Build history of the part. All positions in model axes, mm. Face numbers are marked on the shaded views. A direction names the side the tool comes from. Round coordinates to 2 decimals unless told otherwise and drop trailing zeros. Loops run counter-clockwise (first coordinate to the right, second up) from the corner with the lowest first, then second, coordinate; pieces in that order, holes last. Notation, with made-up numbers: (-9, 9) -> (11, 9) arc R26 ccw to (11, 42) -> close; hole circle Ø11 at (-8.5, 78). An arc over 180 degrees is marked (long way). Put each result on its own line as item: value. Start each with the question number.
Item 1: Drill centre lines: probe 1 along Z at (x, y) = (2.25, 2); probe 2 along Y at (x, z) = (5.25, -16); probe 3 along Y at (x, z) = (5.5, -8). Where is each one in solid material? Low to high. Write a range as [from, to].
Item 2: Cut at D-D, the plane z = 0. List the corners of the cut face in (x, y) (3 decimals).
Item 3: Pull direction Z, two halves, no side cores. Call the marked faces 1, 2 and 3: +Z half, -Z half, draft (parallel to the pull), parting line (faces both ways), or undercut.
Item 4: Cut at A-A, the plane y = 0. List the corners of the cut face in (x, z) (3 decimals).
Item 5: Cut at B-B, the plane z = 9. List the corners of the cut face in (x, y) (3 decimals).
Item 6: Cut at C-C, the plane x = 13.75. List the corners of the cut face in (y, z), plus the area to 3 significant figures.
Item 7: Flat gauge pins, fed straight in: pin 1 Ø9 at (y, z) = (18.02, -17.38) entering from +X (3 decimals); pin 2 Ø11 at (y, z) = (-18.51, 18.23) entering from -X; pin 3 Ø12 at (y, z) = (-20.5, -18.5) entering from +X (3 decimals). Where does each tip first touch, or does it go through?
Item 8: Tool access for the marked faces 4 and 5: list every direction of +Z, -Z, +X, -X, +Y, -Y with a clear straight run to the whole face (end or side of a thin tool).
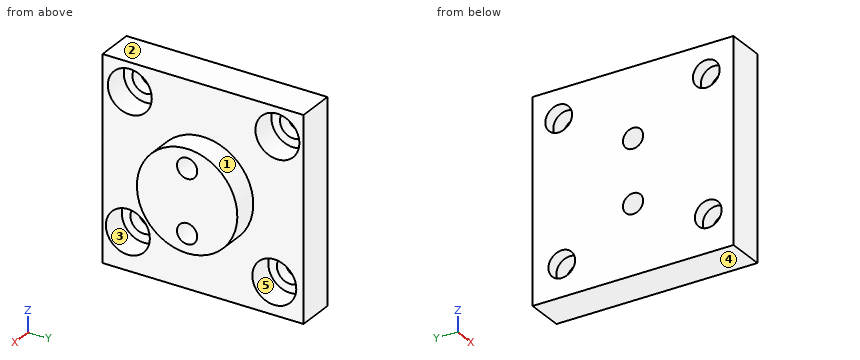
```python
from build123d import *

# Parameters (mm, degrees)
SKETCH1_W                                        = 50.8
SKETCH1_H                                        = 50.8
BOSS_EXTRUDE1_DEPTH                              = 9.525
SKETCH2_R                                        = 12.7
BOSS_EXTRUDE2_DEPTH                              = 6.35
F_1_4_20_TAPPED_HOLE1_D                          = 5.1054
CBORE_FOR_1_4_SOCKET_HEAD_CAP_SCREW1_D           = 6.7564
CBORE_FOR_1_4_SOCKET_HEAD_CAP_SCREW1_CBORE_D     = 11.1125
CBORE_FOR_1_4_SOCKET_HEAD_CAP_SCREW1_CBORE_DEPTH = 6.35


with BuildPart() as part:
    # Sketch1 → Boss-Extrude1 (new body)
    with BuildSketch(Plane(origin=(0, 0, 0), x_dir=(0, 0, -1), z_dir=(1, 0, 0))):
        Rectangle(SKETCH1_W, SKETCH1_H)
    extrude(amount=BOSS_EXTRUDE1_DEPTH)

    # Sketch2 → Boss-Extrude2 (add)
    with BuildSketch(Plane(origin=(9.525, 0, 0), x_dir=(0, 0, -1), z_dir=(1, 0, 0))):
        Circle(SKETCH2_R)
    extrude(amount=BOSS_EXTRUDE2_DEPTH)

    # 1/4-20 Tapped Hole1 (through all)
    with Locations(Plane(origin=(15.875, 0, 0), x_dir=(0, 0, -1), z_dir=(1, 0, 0))):
        with Locations((-7.9375, 0), (7.9375, 0)):
            Hole(F_1_4_20_TAPPED_HOLE1_D / 2)

    # CBORE for 1/4 Socket Head Cap Screw1 (through all)
    with Locations(Plane(origin=(9.525, 0, 0), x_dir=(0, 0, -1), z_dir=(1, 0, 0))):
        with Locations((-18.22919312, 18.79663882), (17.378024569, 18.016400982), (15.959410319, -19.009430957), (-18.22919312, -18.51291597)):
            CounterBoreHole(CBORE_FOR_1_4_SOCKET_HEAD_CAP_SCREW1_D / 2, CBORE_FOR_1_4_SOCKET_HEAD_CAP_SCREW1_CBORE_D / 2, CBORE_FOR_1_4_SOCKET_HEAD_CAP_SCREW1_CBORE_DEPTH)


solid = part.part
```
Reply:
1. probe 1: z = [-25.4, -9.52], [-6.35, 6.35], [9.52, 25.4]
1. probe 2: y = [-25.4, -24.57], [-13.45, 12.63], [23.4, 25.4]
1. probe 3: y = [-25.4, -2.55], [2.55, 25.4]
2. outline: (0, -25.4) -> (9.525, -25.4) -> (9.525, -12.7) -> (15.875, -12.7) -> (15.875, 12.7) -> (9.525, 12.7) -> (9.525, 25.4) -> (0, 25.4) -> close
3. face 1: parting line
3. face 2: +Z half
3. face 3: undercut
4. outline: (0, -25.4) -> (9.525, -25.4) -> (9.525, -12.7) -> (15.875, -12.7) -> (15.875, -10.49) -> (0, -10.49) -> close; (0, -5.385) -> (15.875, -5.385) -> (15.875, 5.385) -> (0, 5.385) -> close; (0, 10.49) -> (15.875, 10.49) -> (15.875, 12.7) -> (9.525, 12.7) -> (9.525, 25.4) -> (0, 25.4) -> close
5. outline: (0, -25.4) -> (9.525, -25.4) -> (9.525, -8.96) -> (15.875, -8.96) -> (15.875, -2.321) -> (0, -2.321) -> close; (0, 2.321) -> (15.875, 2.321) -> (15.875, 8.96) -> (9.525, 8.96) -> (9.525, 25.4) -> (0, 25.4) -> close
6. outline: circle Ø25.4 at (0, 0); hole circle Ø5.11 at (0, -7.94); hole circle Ø5.11 at (0, 7.94)
6. area: 466 mm^2
7. pin 1: stops at x = 3.175
7. pin 2: stops at x = 0
7. pin 3: stops at x = 9.525
8. face 4: -Z, +X, -X, +Y, -Y
8. face 5: +X
